Build history of the part. All positions in model axes, mm. Round coordinates to 2 decimals unless told otherwise and drop trailing zeros. Loops run counter-clockwise (first coordinate to the right, second up) from the corner with the lowest first, then second, coordinate; pieces in that order, holes last.
Autodesk Inventor part; units mm, degrees
ref_plane "YZ Plane" through (0, 0, 0) normal (1, 0, 0) x (0, 1, 0)
ref_plane "XZ Plane" through (0, 0, 0) normal (0, 1, 0) x (-1, 0, 0)
ref_plane "XY Plane" through (0, 0, 0) normal (0, 0, 1) x (1, 0, 0)
sketch "Sketch1" plane through (0, 0, 0) normal (0, 1, 0) x (-1, 0, 0)
  circle A0 centre (0, 0) radius 1
  dimension "d0" = 2
extrude "Extrusion1" add sketch "Sketch1" along normal blind 55
move faces "Move1" translate (0, -2.5, 0) faces at (-0.5848, 55, -0.397)
move faces "Move2" translate (0, -0.002, 0) faces at (-0.2495, 52.5, 0.221)
move faces "Move3" translate (0, -1.862, 0) faces at (-0.2495, 52.498, 0.221)
properties part number "LOOP2_COLL_L"
(1) Slice it at C-C on x = 0.4. List the corners of the cut face in (y, z).
Responses:
outline: (0, -0.92) - (50.64, -0.92) - (50.64, 0.92) - (0, 0.92) - close
(2) Slice it at B-B on z = -0.6. List the corners of the cut face in (x, y), plus the area to 3 significant figures.
Responses:
outline: (-0.8, 0) - (0.8, 0) - (0.8, 50.64) - (-0.8, 50.64) - close
area: 81.0 mm2
(3) Slice it at A-A on y = 47. List the corners of the cut face in (x, z).
Responses:
outline: circle Ø2 at (0, 0)
(4) Probe line 1 (X direction, y = 8, z = -0.8); line 2 (X direction, y = 33.5, z = -0.35); line 3 (Z direction, x = 0.3, y = 2). List the from-to ranges inside material, lowest first.
Responses:
line 1: x = -0.6 to 0.6
line 2: x = -0.94 to 0.94
line 3: z = -0.95 to 0.95
